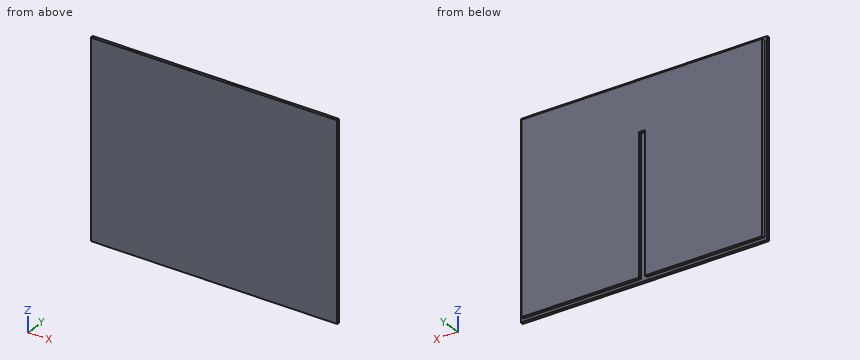
Autodesk Inventor part; units mm, degrees
ref_plane "YZ Plane" through (0, 0, 0) normal (1, 0, 0) x (0, 1, 0)
ref_plane "XZ Plane" through (0, 0, 0) normal (0, 1, 0) x (-1, 0, 0)
ref_plane "XY Plane" through (0, 0, 0) normal (0, 0, 1) x (1, 0, 0)
sketch "Sketch1" plane through (0, 0, 0) normal (0, 1, 0) x (-1, 0, 0)
  line L0 (367.8783, -267.593) -> (-432.2217, -267.593)
  line L1 (-432.2217, -267.593) -> (-432.2217, 354.707)
  line L2 (-432.2217, 354.707) -> (367.8783, 354.707)
  line L3 (367.8783, 354.707) -> (367.8783, -267.593)
  point P0 (0, 0)
  dimension "d0" = 622.3
  dimension "d1" = 800.1
extrude "Board" add sketch "Sketch1" along normal blind 19.05
sketch "Sketch3" plane through (0, 19.05, 0) normal (0, 1, 0) x (1, 0, 0)
  line L0 (432.2217, -354.707) -> (432.2217, 267.593)
  line L1 (22.6467, -186.432) -> (41.6967, -186.432)
  line L2 (41.6967, -186.432) -> (41.6967, 267.593)
  line L3 (41.6967, 267.593) -> (22.6467, 267.593)
  line L4 (22.6467, 267.593) -> (22.6467, -186.432)
  line L5 (432.2217, 267.593) -> (-367.8783, 267.593)
  line L6 (-367.8783, 267.593) -> (-367.8783, -354.707)
  point P0 (0, 0)
  dimension "d17" = 19.05
  dimension "d26" = 454.025
  dimension "d27" = 390.525
extrude "Vertical Wall Dado Cuts" cut sketch "Sketch3" against normal blind 9.525
sketch "Sketch5" plane through (0, 19.05, 0) normal (0, 1, 0) x (1, 0, 0)
  line L0 (-367.8783, -354.707) -> (432.2217, -354.707)
  line L1 (432.2217, -354.707) -> (422.6967, -354.707)
  line L2 (422.6967, -354.707) -> (422.6967, 267.593)
  line L3 (422.6967, 267.593) -> (432.2217, 267.593)
  line L4 (432.2217, 267.593) -> (432.2217, -354.707)
  line L5 (432.2217, 267.593) -> (-367.8783, 267.593)
  line L6 (-367.8783, -354.707) -> (-358.3533, -354.707)
  line L7 (-358.3533, -354.707) -> (-358.3533, 267.593)
  line L8 (-358.3533, 267.593) -> (-367.8783, 267.593)
  line L9 (-367.8783, 267.593) -> (-367.8783, -354.707)
  line L10 (432.2217, 267.593) -> (-367.8783, 267.593)
  line L11 (432.2217, -354.707) -> (-367.8783, -354.707)
  line L12 (-367.8783, -354.707) -> (-367.8783, -345.182)
  line L13 (-367.8783, -345.182) -> (432.2217, -345.182)
  line L14 (432.2217, -345.182) -> (432.2217, -354.707)
  line L15 (-367.8783, 267.593) -> (432.2217, 267.593)
  line L16 (432.2217, 267.593) -> (432.2217, 258.068)
  line L17 (432.2217, 258.068) -> (-367.8783, 258.068)
  line L18 (-367.8783, 258.068) -> (-367.8783, 267.593)
  line L19 (432.2217, -354.707) -> (432.2217, 267.593)
  point P0 (0, 0)
  point P1 (422.6967, 267.593)
  point P2 (22.6467, 267.593)
  point P3 (-348.8283, 267.593)
  dimension "d22" = 9.525
extrude "Perimeter rabbit dado" cut sketch "Sketch5" against normal blind 9.525 contours L9 L13 L7 L0 | L7 L13 L2 L0 | L9 L17 L7 L13 | L2 L13 L4 L0 | L9 L5 L7 L17 | L2 L17 L4 L13 | L7 L5 L2 L17 | L2 L3 L4 L17
equation "\"d27\" = -0.5 * d17 + 0.5 * d1"
properties part number "Top"
Read the model definition and answer for the solid it produces. Units are mm, in the model's axes. Give positions to 0.01 mm unless a question says otherwise; leave off trailing zeros. Order: outer loops, then holes, each group sorted by start corner. A loop starts at its lowest first (then second) coordinate and runs counter-clockwise, first axis right, second up.
(1) Find section C-C (x = -105). Give the vertices of the cut face in (y, z) (3 decimals), plus the area to 3 significant figures.
(2) Given pin 1 (7.5 mm diameter, centred on y = 16.5, z = 46, fed in from -X); pin 2 (7.5 mm diameter, centred on x = -209.5, y = 15, fed in from -Z); pin 3 (5 mm diameter, centred on y = 15.5, z = 186, fed in from +X), each flat-ended and moving along its own axis, determine where each tip first touches the part or whether it passes through.
(3) Straight lines are drawn through the part: L1, parallel to X at y = 9.75, z = -8; L2, parallel to Z at x = 137.5, y = 11.25; L3, parallel to X at y = 12.5, z = 242.5. For each, find the intervals that lie inside material, in ascending order.
(4) Find section A-A (y = 13.25). Give the vertices of the cut face in (x, z), plus the area to 3 significant figures.
(5) Find section B-B (z = 151.5). Give the vertices of the cut face in (x, y) (3 decimals), plus the area to 3 significant figures.
Result sheet:
1. outline: (0, -267.593) - (9.525, -267.593) - (9.525, -258.068) - (19.05, -258.068) - (19.05, 345.182) - (9.525, 345.182) - (9.525, 354.707) - (0, 354.707) - close
1. area: 11,700 mm2
2. pin 1: stops at x = -358.35
2. pin 2: stops at z = -258.07
2. pin 3: stops at x = 422.7
3. L1: x = -358.35 to 22.65, 41.7 to 422.7
3. L2: z = -258.07 to 345.18
3. L3: x = -358.35 to 422.7
4. outline: (-358.35, -258.07) - (22.65, -258.07) - (22.65, 186.43) - (41.7, 186.43) - (41.7, -258.07) - (422.7, -258.07) - (422.7, 345.18) - (-358.35, 345.18) - close
4. area: 463,000 mm2
5. outline: (-367.878, 0) - (432.222, 0) - (432.222, 9.525) - (422.697, 9.525) - (422.697, 19.05) - (41.697, 19.05) - (41.697, 9.525) - (22.647, 9.525) - (22.647, 19.05) - (-358.353, 19.05) - (-358.353, 9.525) - (-367.878, 9.525) - close
5. area: 14,900 mm2
